Autodesk Inventor part; units mm, degrees
ref_plane "YZ Plane" through (0, 0, 0) normal (1, 0, 0) x (0, 1, 0)
ref_plane "XZ Plane" through (0, 0, 0) normal (0, 1, 0) x (-1, 0, 0)
ref_plane "XY Plane" through (0, 0, 0) normal (0, 0, 1) x (1, 0, 0)
sketch "Sketch1" plane through (0, 0, 0) normal (0, 0, 1) x (1, 0, 0)
  line L0 (0, 0) -> (0, 38.1)
  line L1 (0, 38.1) -> (3.175, 38.1)
  line L2 (3.175, 38.1) -> (3.175, 3.175)
  line L3 (3.175, 3.175) -> (38.1, 3.175)
  line L4 (38.1, 3.175) -> (38.1, 0)
  line L5 (38.1, 0) -> (0, 0)
  dimension "d0" = 38.1
  dimension "d1" = 3.175
extrude "Extrusion1" add sketch "Sketch1" along normal blind 485.775
sketch "Sketch4" plane through (3.175, 3.175, 0) normal (1, 0, 0) x (0, 0, -1)
  line L0 (0, 0) -> (-485.775, 0)
  line L1 (0, -3.175) -> (0, 34.925)
  line L2 (0, 34.925) -> (-26.0631, -10.2176)
  line L3 (-26.0631, -10.2176) -> (14.7874, -10.2176)
  line L4 (14.7874, -10.2176) -> (14.7874, 34.925)
  line L5 (14.7874, 34.925) -> (0, 34.925)
  line L6 (-20.164, 0) -> (29.2522, 0)
  dimension "d6" = 60
extrude "Extrusion2" cut sketch "Sketch4" along normal mid plane 476.25
sketch "Sketch5" plane through (3.175, 3.175, 485.775) normal (1, 0, 0) x (0, 0, -1)
  line L0 (0, 0) -> (0, 34.925)
  line L1 (465.611, 0) -> (0, 0)
  line L2 (465.611, 0) -> (485.775, 34.925)
  line L3 (485.775, 34.925) -> (0, 34.925)
  line L4 (471.1103, 34.925) -> (450.9463, 0)
  point P0 (485.775, -3.175)
  point P1 (19.05, 19.05)
  point P2 (461.9449, 19.05)
  dimension "d9" = 19.05
  dimension "d10" = 19.05
  dimension "d11" = 12.7
hole "Hole1" at (3.175, 22.225, 466.725) at (3.175, 22.225, 23.8301) direction (-1, 0, 0) diameter 9.525 end through all
sketch "Sketch6" plane through (3.175, 3.175, 485.775) normal (0, 1, 0) x (1, 0, 0)
  line L0 (0, 485.775) -> (0, 0)
  line L1 (34.925, 0) -> (0, 0)
  line L2 (34.925, 465.611) -> (34.925, 0)
  point P0 (-3.175, 485.775)
  point P1 (23.3172, 34.7472)
  point P2 (8.9154, 19.4564)
  dimension "d20" = 8.9154
  dimension "d21" = 19.4564
  dimension "d22" = 11.6078
  dimension "d23" = 34.7472
hole "Hole2" at (26.4922, 3.175, 451.0278) at (12.0904, 3.175, 466.3186) direction (0, -1, 0) diameter 5.1054 end through all
sketch "Sketch7" plane through (3.175, 3.175, 485.775) normal (1, 0, 0) x (0, 0, -1)
  circle A0 centre (19.05, 19.05) radius 4.7625
  line L0 (0, 0) -> (0, 34.925)
  point P0 (485.775, -3.175)
  point P1 (190.5, 19.05)
  point P2 (247.65, 19.05)
  point P3 (304.8, 19.05)
  point P4 (361.95, 19.05)
  point P5 (419.1, 19.05)
  dimension "d31" = 190.5
  dimension "d32" = 57.15
  dimension "d35" = 57.15
  dimension "d45" = 57.15
  dimension "d46" = 57.15
hole "Hole3" at (3.175, 22.225, 295.275) at (3.175, 22.225, 238.125) at (3.175, 22.225, 180.975) at (3.175, 22.225, 123.825) at (3.175, 22.225, 66.675) direction (-1, 0, 0) diameter 5.1054 end through all
properties part number "CLB_084_ClimberMountTopAngle" material "Aluminum 6061"
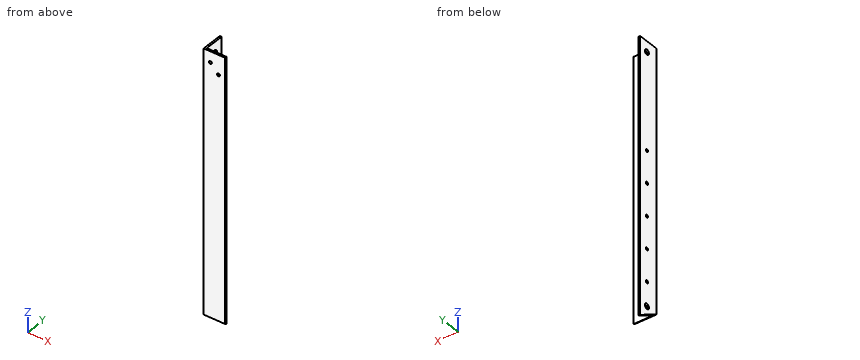
Input: part model. Units: mm. Frame: model coordinates. Give positions to 0.01 mm unless a question says otherwise; leave off trailing zeros. Loops run counter-clockwise (first coordinate to the right, second up) from the corner with the lowest first, then second, coordinate; pieces in that order, holes last. Notation, with made-up numbers: (48, -12.5) -> (72, -12.5) arc R18 ccw to (72, 6.5) -> close; hole circle Ø11 at (86.5, -1). An arc over 180 degrees is marked (long way). Use a Markdown table: item, result.
Q1. First-contact query: P1, Ø8, axis at y = 22.225, z = 66.675, coming from the -X side; P2, Ø5, axis at y = 8, z = 435, coming from the +X side (3 decimals); P3, Ø3, axis at x = 14.5, z = 421, coming from the +Y side (3 decimals). Flat tips, straight axial feed; report the tip coordinate or a pass-through.
Entries:
| item | result |
|---|---|
| P1 | stops at x = 0 |
| P2 | stops at x = 3.175 |
| P3 | stops at y = 3.175 |
Q2. Section query B-B, the plane x = 34. Return the cut outline in (y, z) (3 decimals), plus the area to 3 significant figures.
Entries:
| item | result |
|---|---|
| outline | (0, 21.997) -> (3.175, 20.164) -> (3.175, 485.775) -> (0, 485.775) -> close |
| area | 1,480 mm² |
Q3. Ray query, probe 1 along Y at (x, z) = (14, 164.5) (3 decimals). Return the intervals inside material, ascending. Write a range as from..to.
Entries:
| item | result |
|---|---|
| probe 1 | y = 0..3.175 |
Q4. Section query A-A, the plane z = 311. Return the cut outline in (x, y) (3 decimals).
Entries:
| item | result |
|---|---|
| outline | (0, 0) -> (38.1, 0) -> (38.1, 3.175) -> (3.175, 3.175) -> (3.175, 38.1) -> (0, 38.1) -> close |
